Geometry check sheet. Reference: the model listing, model coordinates, mm. Round coordinates to 2 decimals unless told otherwise and drop trailing zeros. Order: outer loops, then holes, each group sorted by start corner. A loop starts at its lowest first (then second) coordinate and runs counter-clockwise, first axis right, second up. Notation, with made-up numbers: (-9.5, 88) - (37.5, 88) arc R22 ccw to (37.5, 103) - close; hole circle Ø11 at (62.25, 2). An arc over 180 degrees is marked (long way). Return JSON: item names as keys, results as strings. Group by question number.
Q1. Draft check along Z on faces 1 (the flat face through (1, -3.175, 2)), 2 (the cylindrical face through (-71.01, -1.61, -93.915)), 3 (the cylindrical face through (-98.884, -1.61, -140.011)), 4 (the cylindrical face through (98.884, -1.61, 140.011)). Enter one of: pulls with the +Z half, pulls with the -Z half, needs draft (parallel to the pull), parting line crosses it, or undercut.
Q2. Sectioned sample at A-A, the plane x = 63.5. Record the cut outline in (y, z) (1 decimal).
Q3. Material ranges on line 1 along Z through (x, y) = (63.5, -1.9) (1 decimal); line 2 along Z through (x, y) = (58.5, -2.25) (3 decimals); line 3 along X through (y, z) = (-1.05, -92.5), recorded low to high.
Q4. Sectioned sample at C-C, the plane x = -56. Record the cut outline in (y, z) (3 decimals).
Q5. Sectioned sample at B-B, the plane y = -1.65. Give the number of separate pieces and of enclosed holes in the cut face, then the cut area to 3 significant figures.
Autodesk Inventor part; units mm, degrees
ref_plane "YZ Plane" through (0, 0, 0) normal (1, 0, 0) x (0, 1, 0)
ref_plane "XZ Plane" through (0, 0, 0) normal (0, 1, 0) x (-1, 0, 0)
ref_plane "XY Plane" through (0, 0, 0) normal (0, 0, 1) x (1, 0, 0)
sketch "Sketch1" plane through (0, 0, 0) normal (0, 1, 0) x (-1, 0, 0)
  line L0 (101.6, -142.875) -> (-101.6, -142.875)
  line L1 (-101.6, -142.875) -> (-101.6, 142.875)
  line L2 (-101.6, 142.875) -> (101.6, 142.875)
  line L3 (101.6, 142.875) -> (101.6, -142.875)
  line L4 (101.6, -142.875) -> (-101.6, 142.875) construction
  line L5 (-101.6, -142.875) -> (101.6, 142.875) construction
  point P0 (0, 0)
  dimension "d0" = 203.2
  dimension "d1" = 285.75
extrude "Extrusion1" add sketch "Sketch1" against normal blind 3.175
sketch "Sketch2" plane through (0, 0, 0) normal (0, 1, 0) x (1, 0, 0)
  line L0 (101.6, 142.875) -> (101.6, -142.875) construction
  line L1 (101.6, 0) -> (-101.6, 0) construction
  line L2 (-101.6, -142.875) -> (-101.6, 142.875) construction
  line L3 (-101.6, 142.875) -> (101.6, 142.875) construction
  line L4 (0, 142.875) -> (0, -142.875) construction
  point P0 (0, 0)
  point P1 (63.5, 85.725)
  point P2 (0, 0)
  point P3 (-63.5, 85.725)
  point P4 (63.5, -85.725)
  point P5 (-63.5, -85.725)
  point P6 (0, 0)
  dimension "d4" = 85.725
  dimension "d5" = 63.5
hole "Hole1" at (63.5, 0, -85.725) at (-63.5, 0, -85.725) at (63.5, 0, 85.725) at (-63.5, 0, 85.725) direction (0, -1, 0) diameter 22.225 end through all
fillet "Fillet1" radius 9.525 4 edges at (101.6, -1.5875, 142.875) (101.6, -1.5875, -142.875) (-101.6, -1.5875, 142.875) (-101.6, -1.5875, -142.875)
properties part number "GP2-001" material "Aluminum 6061"
Reply:
{
 "1": {"face 1": "needs draft", "face 2": "undercut", "face 3": "pulls with the -Z half", "face 4": "pulls with the +Z half"},
 "2": {"outline": "(-3.2, -142.9) - (0, -142.9) - (0, -96.8) - (-3.2, -96.8) - close; (-3.2, -74.6) - (0, -74.6) - (0, 74.6) - (-3.2, 74.6) - close; (-3.2, 96.8) - (0, 96.8) - (0, 142.9) - (-3.2, 142.9) - close"},
 "3": {"line 1": "-142.9 to -96.8, -74.6 to 74.6, 96.8 to 142.9", "line 2": "-142.875 to -95.649, -75.801 to 75.801, 95.649 to 142.875", "line 3": "-101.6 to -72.31, -54.69 to 54.69, 72.31 to 101.6"},
 "4": {"outline": "(-3.175, -142.875) - (0, -142.875) - (0, -93.925) - (-3.175, -93.925) - close; (-3.175, -77.525) - (0, -77.525) - (0, 77.525) - (-3.175, 77.525) - close; (-3.175, 93.925) - (0, 93.925) - (0, 142.875) - (-3.175, 142.875) - close"},
 "5": {"separate pieces": "1", "enclosed holes": "4", "area": "56,400 mm^2"}
}
